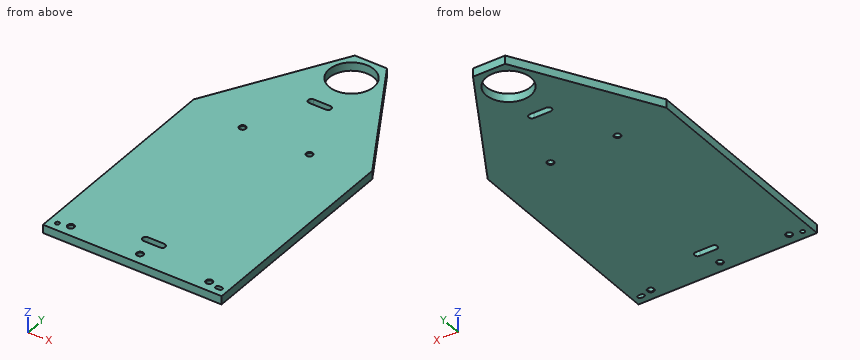
from build123d import *

# Parameters (mm, degrees)
SKETCH6_R                        = 25.4
BOSS_EXTRUDE1_DEPTH              = 4.7625
F_1_4_20_TAPPED_HOLE1_AT_2_COUNT = 2
F_1_4_20_TAPPED_HOLE1_AT_2_PITCH = 76.2
F_3_16_0_1875_DIAMETER_HOLE1_D   = 4.7752
CUT_EXTRUDE1_DEPTH               = 10.525
F_1_4_20_TAPPED_HOLE2_AT_2_COUNT = 2
F_1_4_20_TAPPED_HOLE2_AT_2_PITCH = 78.74
F_1_4_20_TAPPED_HOLE2_AT_3_COUNT = 2
F_1_4_20_TAPPED_HOLE2_AT_3_PITCH = 78.74


with BuildPart() as part:
    # Sketch6 → Boss-Extrude1 (new body, symmetric)
    with BuildSketch(Plane.XY):
        Polygon((-101.6, 0), (101.6, 0), (101.6, 247.225737951), (18.330871047, 391.4521), (-18.330871047, 391.4521), (-101.6, 247.225737951), align=None)
        with Locations((0, 359.7021)):
            Circle(SKETCH6_R, mode=Mode.SUBTRACT)
        with BuildLine():
            Line((9.525, 31.9913), (-9.525, 31.9913))
            ThreePointArc((-9.525, 31.9913), (-13.0937, 35.56), (-9.525, 39.1287))
            Line((-9.525, 39.1287), (9.525, 39.1287))
            ThreePointArc((9.525, 39.1287), (13.0937, 35.56), (9.525, 31.9913))
        make_face(mode=Mode.SUBTRACT)
        with BuildLine():
            Line((9.525, 304.0253), (-9.525, 304.0253))
            ThreePointArc((-9.525, 304.0253), (-13.0937, 307.594), (-9.525, 311.1627))
            Line((-9.525, 311.1627), (9.525, 311.1627))
            ThreePointArc((9.525, 311.1627), (13.0937, 307.594), (9.525, 304.0253))
        make_face(mode=Mode.SUBTRACT)
    extrude(amount=BOSS_EXTRUDE1_DEPTH, both=True)

    # Sketch7 → 1/4-20 Tapped Hole1 (revolve, cut)
    with BuildSketch(Plane(origin=(-38.1, 235.8771, 4.7625), x_dir=(0, -1, 0), z_dir=(1, 0, 0))):
        Polygon((0, 0), (0, 9.525), (3.81, 9.525), (3.175, 8.89), (3.175, 0.635), (3.81, 0), align=None)
    f_1_4_20_tapped_hole1 = revolve(axis=Axis((-38.1, 235.8771, 11.1125), (0, 0, -1)), mode=Mode.SUBTRACT)

    # 1/4-20 Tapped Hole1 at 2: 1/4-20 Tapped Hole1 ×2
    with Locations(*[(i * F_1_4_20_TAPPED_HOLE1_AT_2_PITCH, 0, 0) for i in range(1, F_1_4_20_TAPPED_HOLE1_AT_2_COUNT)]):
        add(f_1_4_20_tapped_hole1, mode=Mode.SUBTRACT)

    # 3/16 (0.1875) Diameter Hole1 (through all)
    with Locations(Plane(origin=(643.650137784, 199.419465463, 4.7625), x_dir=(1, 0, 0), z_dir=(0, 0, 1))):
        with Locations((-735.598137784, -189.767465463)):
            Hole(F_3_16_0_1875_DIAMETER_HOLE1_D / 2)

    # Sketch13 → Cut-Extrude1 (cut, through all)
    with BuildSketch(Plane.XY.offset(4.7625)):
        with BuildLine():
            Line((90.424, 12.0396), (93.472, 12.0396))
            ThreePointArc((93.472, 12.0396), (95.8596, 9.652), (93.472, 7.2644))
            Line((93.472, 7.2644), (90.424, 7.2644))
            ThreePointArc((90.424, 7.2644), (88.0364, 9.652), (90.424, 12.0396))
        make_face()
    extrude(amount=-CUT_EXTRUDE1_DEPTH, mode=Mode.SUBTRACT)

    # Sketch11 → 1/4-20 Tapped Hole2 (revolve, cut)
    with BuildSketch(Plane(origin=(0, 12.7, 4.7625), x_dir=(0, -1, 0), z_dir=(1, 0, 0))):
        Polygon((0, 0), (0, 9.525), (3.81, 9.525), (3.175, 8.89), (3.175, 0.635), (3.81, 0), align=None)
    f_1_4_20_tapped_hole2 = revolve(axis=Axis((0, 12.7, 11.1125), (0, 0, -1)), mode=Mode.SUBTRACT)

    # 1/4-20 Tapped Hole2 at 2: 1/4-20 Tapped Hole2 ×2
    with Locations(*[(i * F_1_4_20_TAPPED_HOLE2_AT_2_PITCH, 0, 0) for i in range(1, F_1_4_20_TAPPED_HOLE2_AT_2_COUNT)]):
        add(f_1_4_20_tapped_hole2, mode=Mode.SUBTRACT)

    # 1/4-20 Tapped Hole2 at 3: 1/4-20 Tapped Hole2 ×2
    with Locations(*[(-i * F_1_4_20_TAPPED_HOLE2_AT_3_PITCH, 0, 0) for i in range(1, F_1_4_20_TAPPED_HOLE2_AT_3_COUNT)]):
        add(f_1_4_20_tapped_hole2, mode=Mode.SUBTRACT)


solid = part.part
The model under review builds one solid part; all positions refer to its coordinate system, in mm. Coordinates: 2 decimals unless noted, no trailing zeros. Write each loop counter-clockwise with the first axis right and the second up, starting at its lowest first coordinate (ties: lowest second). Pieces come first, ordered by that corner, then holes. Notation, with made-up numbers: M 61.25,88.5 L 72.25,88.5 A34 cw 72.25,120.5 Z; hole C 17.5,-1.5 d6. An arc over 180 degrees is marked long. Put each result on its own line as item: value.
1) Wall thickness on probe 1 along X at (y, z) = (12.7, 2.25) (3 decimals); probe 2 along Y at (x, z) = (0, 0.75) (3 decimals); probe 3 along Y at (x, z) = (-2, -2.5): over which ranges is each line inside the solid? List them lowest first. Write a range as [from, to].
Computed:
probe 1: x = [-101.6, -81.915], [-75.565, -3.175], [3.175, 75.565], [81.915, 101.6]
probe 2: y = [0, 9.525], [15.875, 31.991], [39.129, 304.025], [311.163, 334.302], [385.102, 391.452]
probe 3: y = [0, 10.23], [15.17, 31.99], [39.13, 304.03], [311.16, 334.38], [385.02, 391.45]
2) Add section B-B on z = -1.75. State how many separate pieces and enclosed holes the cut face has, then the cut area to 3 significant figures.
Computed:
separate pieces: 1
enclosed holes: 10
area: 64,900 mm2
3) Clearance check with flat-ended pins moving along their axes: pin 1 Ø4 at (x, y) = (0, 12.7) entering from -Z; pin 2 Ø3.5 at (x, z) = (92, 0.5) entering from +Y. State where each tip first meets the part, or that it passes through.
Computed:
pin 1: passes through
pin 2: stops at y = 266.88
4) Add section A-A on y = 35.56. Give the boundary of the cut face in (x, z).
Computed:
outline: M -101.6,-4.76 L -13.09,-4.76 L -13.09,4.76 L -101.6,4.76 Z; M 13.09,-4.76 L 101.6,-4.76 L 101.6,4.76 L 13.09,4.76 Z
